Input: part model. Units: mm. Frame: model coordinates. Coordinates: 2 decimals unless noted, no trailing zeros. Order: outer loops, then holes, each group sorted by start corner. A loop starts at its lowest first (then second) coordinate and runs counter-clockwise, first axis right, second up. Notation, with made-up numbers: M 28.5,5.5 L 33.5,5.5 A32 cw 33.5,37.5 Z; hole C 66,-35.5 d1. An arc over 180 degrees is marked long. One line per item, written item: value.
```python
from build123d import *

# Parameters (mm, degrees)
SKETCH1_R           = 50.8
SKETCH1_R_2         = 2
BOSS_EXTRUDE1_DEPTH = 5.842
CHAMFER1_SIZE       = 2.3


with BuildPart() as part:
    # Sketch1 → Boss-Extrude1 (new body)
    with BuildSketch(Plane(origin=(0, 0, 0), x_dir=(1, 0, 0), z_dir=(0, 1, 0))):
        Circle(SKETCH1_R)
        with Locations((-25.4, 25.4)):
            Circle(SKETCH1_R_2, mode=Mode.SUBTRACT)
        with Locations((25.4, 25.4)):
            Circle(SKETCH1_R_2, mode=Mode.SUBTRACT)
        with Locations((25.4, -25.4)):
            Circle(SKETCH1_R_2, mode=Mode.SUBTRACT)
        with Locations((-25.4, -25.4)):
            Circle(SKETCH1_R_2, mode=Mode.SUBTRACT)
    extrude(amount=BOSS_EXTRUDE1_DEPTH)

    # Chamfer1
    chamfer1_edges = [part.edges().sort_by_distance(p)[0] for p in [
        (23.4, 5.842, -25.4),
        (23.4, 5.842, 25.4),
        (-27.4, 5.842, -25.4),
        (-27.4, 5.842, 25.4),
    ]]
    chamfer(chamfer1_edges, length=CHAMFER1_SIZE)


solid = part.part
```
(1) Cut plane B-B on z = 25.4. Output: boundary loops of the cut face in (x, y), plus the area to 3 significant figures.
Data:
outline: M -43.99,0 L -27.4,0 L -27.4,3.54 L -29.7,5.84 L -43.99,5.84 Z; M -23.4,0 L 23.4,0 L 23.4,3.54 L 21.1,5.84 L -21.1,5.84 L -23.4,3.54 Z; M 27.4,0 L 43.99,0 L 43.99,5.84 L 29.7,5.84 L 27.4,3.54 Z
area: 457 mm2
(2) Cut plane D-D on x = 42.5. Output: boundary loops of the cut face in (y, z), plus the area to 3 significant figures.
Data:
outline: M 0,-27.83 L 5.84,-27.83 L 5.84,27.83 L 0,27.83 Z
area: 325 mm2
(3) Draft query along Z for faces 1 (the conical face through (-26.98, 3.686, 23.951)), 2 (the cylindrical face through (-23.553, 1.746, 26.166)), 3 (the flat face through (-1, 0, -1)), 4 (the cylindrical face through (-11.012, 2.88, 49.592)). Return one class per face: released by +Z, released by -Z, zero draft, split by the parting line, or undercut.
Data:
face 1: undercut
face 2: undercut
face 3: zero draft
face 4: split by the parting line
(4) Ray query, line 1 (Z direction, x = -25.4, y = 1.9); line 2 (Z direction, x = -26, y = 1.4). Return the intervals inside material, ascending. Write a range as from..to.
Data:
line 1: z = -43.99..-27.4, -23.4..23.4, 27.4..43.99
line 2: z = -43.64..-27.31, -23.49..23.49, 27.31..43.64
(5) Cut plane A-A on x = -25.4. Output: boundary loops of the cut face in (y, z).
Data:
outline: M 0,-43.99 L 5.84,-43.99 L 5.84,-29.7 L 3.54,-27.4 L 0,-27.4 Z; M 0,-23.4 L 3.54,-23.4 L 5.84,-21.1 L 5.84,21.1 L 3.54,23.4 L 0,23.4 Z; M 0,27.4 L 3.54,27.4 L 5.84,29.7 L 5.84,43.99 L 0,43.99 Z
(6) First-contact query: pin 1 (4.5 mm diameter, centred on x = -25.4, z = 25.4, fed in from +Y); pin 2 (2 mm diameter, centred on y = 3, z = -34, fed in from -X); pin 3 (3 mm diameter, centred on x = 25.4, z = 25.4, fed in from -Y); pin 4 (3 mm diameter, centred on x = 21, y = 2.5, fed in from -Z). Flat tips, straight axial feed; report the tip coordinate or a pass-through.
Data:
pin 1: stops at y = 3.79
pin 2: stops at x = -38.62
pin 3: passes through
pin 4: stops at z = -46.91
(7) Cut plane C-C on y = 2.65. Output: boundary loops of the cut face in (x, z).
Data:
outline: C 0,0 d101.6; hole C -25.4,-25.4 d4; hole C -25.4,25.4 d4; hole C 25.4,-25.4 d4; hole C 25.4,25.4 d4
